from build123d import *

# Parameters (mm, degrees)
F1_DEPTH = 10
F2_R     = 1


with BuildPart() as f1:
    # F0 (on Front) → F1 (new body)
    with BuildSketch(Plane.XZ):
        with BuildLine():
            add(Edge.make_bspline(
                [(-64.7320359031, 5.8960603655), (-123.067537089, -37.923051477), (-50.1862094657, -41.3079215098)],
                knots=[2.3230612235, 2.3230612235, 2.3230612235, 3.9601240836, 3.9601240836, 3.9601240836], degree=2, weights=[1, 0.68329421, 1]))
            ThreePointArc((-50.1862094657, -41.3079215098), (19.1414535528, -62.1176686289), (64.7320359031, -5.8960603655))
            add(Edge.make_bspline(
                [(64.7320359031, -5.8960603655), (123.067537089, 37.923051477), (50.1862094657, 41.3079215098)],
                knots=[5.4646538771, 5.4646538771, 5.4646538771, 7.1017167372, 7.1017167372, 7.1017167372], degree=2, weights=[1, 0.68329421, 1]))
            ThreePointArc((50.1862094657, 41.3079215098), (-19.1414535528, 62.1176686289), (-64.7320359031, 5.8960603655))
        make_face()
        Polygon((-32.1517660584, -23.8230923945), (-30.3628287151, -9.0500386362), (-23.268740969, -22.0387625849), (-8.7588094598, -19.1241582619), (-18.9257184403, -29.9904996859), (-11.9027429034, -42.8490227002), (-25.1687248766, -36.6629937131), (-34.9759067352, -47.1448605899), (-33.2502658453, -32.8945092697), (-46.5162478185, -26.7084802827), align=None, mode=Mode.SUBTRACT)
        Polygon((32.1517660584, -23.8230923945), (46.5162478185, -26.7084802827), (33.2502658453, -32.8945092697), (34.9759067352, -47.1448605899), (25.1687248766, -36.6629937131), (11.9027429034, -42.8490227002), (18.9257184403, -29.9904996859), (8.7588094598, -19.1241582619), (23.268740969, -22.0387625849), (30.3628287151, -9.0500386362), align=None, mode=Mode.SUBTRACT)
        Polygon((-23.268740969, 22.0387625849), (-30.3628287151, 9.0500386362), (-32.1517660584, 23.8230923945), (-46.5162478185, 26.7084802827), (-33.2502658453, 32.8945092697), (-34.9759067352, 47.1448605899), (-25.1687248766, 36.6629937131), (-11.9027429034, 42.8490227002), (-18.9257184403, 29.9904996859), (-8.7588094598, 19.1241582619), align=None, mode=Mode.SUBTRACT)
        Polygon((0, -7.5166247813), (-11.9186989036, -16.2903154078), (-7.2966644485, -2.1453441579), (-19.0958885106, 6.540397666), (-4.4584969281, 6.540397666), (0, 20.1848893888), (4.4584969281, 6.540397666), (19.0958885106, 6.540397666), (7.2966644485, -2.1453441579), (11.9186989036, -16.2903154078), align=None, mode=Mode.SUBTRACT)
        Polygon((25.1687248766, 36.6629937131), (34.9759067352, 47.1448605899), (33.2502658453, 32.8945092697), (46.5162478185, 26.7084802827), (32.1517660584, 23.8230923945), (30.3628287151, 9.0500386362), (23.268740969, 22.0387625849), (8.7588094598, 19.1241582619), (18.9257184403, 29.9904996859), (11.9027429034, 42.8490227002), align=None, mode=Mode.SUBTRACT)
    extrude(amount=F1_DEPTH)

    # F2
    f2_edges = [f1.edges().sort_by_distance(p)[0] for p in [
        (-34.975907, -5, 47.144861),
        (-11.902743, -5, 42.849023),
        (-46.516248, -5, 26.70848),
        (-30.362829, -5, 9.050039),
        (-8.758809, -5, 19.124158),
        (46.516248, -5, 26.70848),
        (30.362829, -5, 9.050039),
        (8.758809, -5, 19.124158),
        (11.902743, -5, 42.849023),
        (34.975907, -5, 47.144861),
        (0, -5, 20.184889),
        (19.095889, -5, 6.540398),
        (-19.095889, -5, 6.540398),
        (11.918699, -5, -16.290315),
        (-11.918699, -5, -16.290315),
        (46.516248, -5, -26.70848),
        (30.362829, -5, -9.050039),
        (34.975907, -5, -47.144861),
        (8.758809, -5, -19.124158),
        (11.902743, -5, -42.849023),
        (-46.516248, -5, -26.70848),
        (-34.975907, -5, -47.144861),
        (-11.902743, -5, -42.849023),
        (-8.758809, -5, -19.124158),
        (-30.362829, -5, -9.050039),
    ]]
    fillet(f2_edges, radius=F2_R)


solid = f1.part
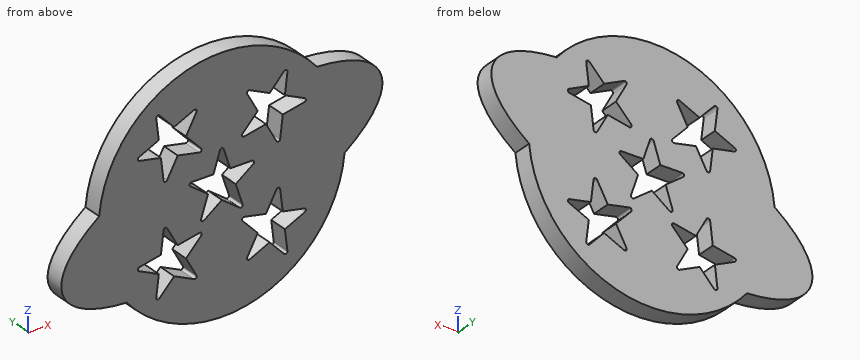
Geometry: final body of the model. Coordinates: model frame, mm. Round coordinates to 2 decimals unless told otherwise and drop trailing zeros. Loops run counter-clockwise (first coordinate to the right, second up) from the corner with the lowest first, then second, coordinate; pieces in that order, holes last. Notation, with made-up numbers: (15, -28) -> (43, -28) arc R32 ccw to (43, 0) -> close; hole circle Ø6 at (44, 52.25). An arc over 180 degrees is marked (long way). One line per question, with ' | ' between items. Start each with the question number.
1. Line query: line 1 along Z through (x, y) = (-28, -2.5); line 2 along X through (y, z) = (-2.25, -44); line 3 along X through (y, z) = (-6.5, 45). Output: solid intervals per line, ascending. Write a range as [from, to].
2. Section A-A on x = -38. Output: boundary loops of the cut face in (y, z).
3. Section B-B on y = -7. Count the separate pieces of the cut face and the enclosed holes in it, and give its area (3 significant figures).
4. Section D-D on z = 55. Output: boundary loops of the cut face in (x, y), and give its area (3 significant figures).
5. Contact query for flat-ended pins moving along their axis: pin 1 (6 mm diameter, centred on x = -36, y = -4.5, fed in from -Z); pin 2 (3 mm diameter, centred on x = -14.5, y = -1.5, fed in from -Z); pin 3 (2 mm diameter, centred on x = 42.5, y = -8.5, fed in from -Z). Output: stop coordinate, or through.
6. Section C-C on z = -52. Output: boundary loops of the cut face in (x, y), and give its area (3 significant figures).
Returned:
1) line 1: z = [-58.66, -39.69], [-13.38, 13.38], [39.69, 58.66] | line 2: x = [-47.84, -34.6], [-32.03, 32.03], [34.6, 47.84] | line 3: x = [-46.9, -34.25], [-32.98, 32.98], [34.25, 46.9]
2) outline: (-10, -52.74) -> (0, -52.74) -> (0, -30.68) -> (-10, -30.68) -> close; (-10, -25) -> (0, -25) -> (0, 25) -> (-10, 25) -> close; (-10, 30.68) -> (0, 30.68) -> (0, 52.74) -> (-10, 52.74) -> close
3) separate pieces: 1 | enclosed holes: 5 | area: 12,600 mm2
4) outline: (-34.64, -10) -> (34.64, -10) -> (34.64, 0) -> (-34.64, 0) -> close | area: 693 mm2
5) pin 1: stops at z = -56 | pin 2: stops at z = -63.69 | pin 3: stops at z = -50.03
6) outline: (-39, -10) -> (39, -10) -> (39, 0) -> (-39, 0) -> close | area: 780 mm2
